```python
from build123d import *

# Parameters (mm, degrees)
SKICA1_W                 = 50
SKICA1_H                 = 50
P_IDAT_VYSUNUT_M2_DEPTH  = 3
SKICA5_W                 = 5
SKICA5_H                 = 22.5
SKICA5_W_2               = 50
SKICA5_H_2               = 5
ODEBRAT_VYSUNUT_M3_DEPTH = 1
P_IDAT_VYSUNUT_M9_DEPTH  = 15
SKICA17_R                = 2
ODEBRAT_VYSUNUT_M8_DEPTH = 4


with BuildPart() as part:
    # Skica1 → Přidat vysunutím2 (new body)
    with BuildSketch(Plane.XY):
        Rectangle(SKICA1_W, SKICA1_H)
    extrude(amount=P_IDAT_VYSUNUT_M2_DEPTH)

    # Skica5 → Odebrat vysunutím3 (cut)
    with BuildSketch(Plane(origin=(0, 0, 0), x_dir=(-1, 0, 0), z_dir=(0, 0, -1))):
        with Locations((0, -13.75)):
            Rectangle(SKICA5_W, SKICA5_H)
        Rectangle(SKICA5_W_2, SKICA5_H_2)
    extrude(amount=-ODEBRAT_VYSUNUT_M3_DEPTH, mode=Mode.SUBTRACT)

    # Skica14 → Přidat vysunutím9 (add)
    with BuildSketch(Plane.XY.offset(3)):
        Polygon((25, 25), (-25, 25), (-25, -25), (-24, -25), (-24, 24), (24, 24), (24, -25), (25, -25), align=None)
    extrude(amount=P_IDAT_VYSUNUT_M9_DEPTH)

    # Skica17 → Odebrat vysunutím8 (cut)
    with BuildSketch(Plane(origin=(0, 0, 1), x_dir=(-1, 0, 0), z_dir=(0, 0, -1))):
        with Locations((-16, 0)):
            Circle(SKICA17_R)
        with Locations((16, 0)):
            Circle(SKICA17_R)
        with Locations((0, -16)):
            Circle(SKICA17_R)
    extrude(amount=-ODEBRAT_VYSUNUT_M8_DEPTH, mode=Mode.SUBTRACT)


solid = part.part
```
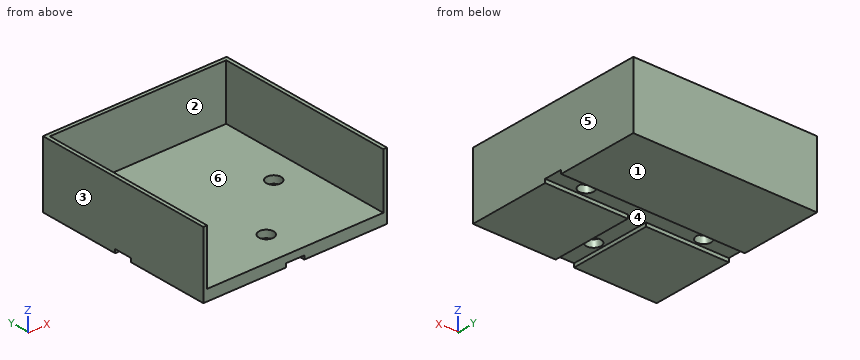
The listing builds one solid part. Answer for the finished solid, in the listing's coordinates (mm). Face numbers are marked on the shaded views. A direction names the side the tool comes from. Give positions to 0.01 mm unless a question says otherwise; leave off trailing zeros. Order: outer loops, then holes, each group sorted by start corner. A loop starts at its lowest first (then second) coordinate and runs counter-clockwise, first axis right, second up. Notation, with made-up numbers: (78.25, -13) -> (105.25, -13) arc R23 cw to (105.25, 19) -> close; hole circle Ø9 at (-6, 34.25). An arc over 180 degrees is marked (long way). Answer as a JSON object with one key per item and string values. Group by question number.
Item 1: Consider L1, parallel to X at y = 6.5, z = 6.5; L2, parallel to Y at x = 16, z = 2.6; L3, parallel to Z at x = 4, y = -2. Determine where each line is inside the solid, lowest interval first. Write a range as from..to.
Item 2: The part is cut by section D-D on y = -16. Write down the section's boundary in (x, z).
Item 3: The part is cut by section A-A on y = 0. Write down the section's boundary in (x, z).
Item 4: Flat-ended cylindrical pins translate along their axes: pin 1 (2 mm diameter, centred on x = 14.5, z = 12.5, fed in from -Y); pin 2 (0.5 mm diameter, centred on x = -1, z = 0.5, fed in from -Y); pin 3 (5 mm diameter, centred on x = 16, y = 0, fed in from +Z). Find the tip coordinate at first contact, or state that the pin passes through.
Item 5: A tool of negligible diameter and unlimited length cuts with its end or side. For the marked faces 1 and 2, from which of +Z, -Z, +X, -X, +Y, -Y can it reach the whole face along a straight path? Write none if from no direction.
Item 6: Determine the mould class of the marked faces 3, 4, 5 and 6 for opening direction X: pulls with the +X half, pulls with the -X half, needs draft (parallel to the pull), parting line crosses it, or undercut.
Item 7: The part is cut by section B-B on x = -16. Write down the section's boundary in (y, z), and give its area (3 significant figures).
Item 8: The part is cut by section C-C on z = 2.25. Write down the section's boundary in (x, y).
Result set:
{
 "1": {"L1": "-25..-24, 24..25", "L2": "-25..-2, 2..25", "L3": "1..3"},
 "2": {"outline": "(-25, 0) -> (-2.5, 0) -> (-2.5, 1) -> (-2, 1) -> (-2, 3) -> (-24, 3) -> (-24, 18) -> (-25, 18) -> close; (2, 1) -> (2.5, 1) -> (2.5, 0) -> (25, 0) -> (25, 18) -> (24, 18) -> (24, 3) -> (2, 3) -> close"},
 "3": {"outline": "(-25, 1) -> (-18, 1) -> (-18, 3) -> (-24, 3) -> (-24, 18) -> (-25, 18) -> close; (-14, 1) -> (14, 1) -> (14, 3) -> (-14, 3) -> close; (18, 1) -> (25, 1) -> (25, 18) -> (24, 18) -> (24, 3) -> (18, 3) -> close"},
 "4": {"pin 1": "y = 24", "pin 2": "y = 2.5", "pin 3": "z = 3"},
 "5": {"face 1": "-Z, +X, -X, +Y, -Y", "face 2": "+Z, -Y"},
 "6": {"face 3": "pulls with the -X half", "face 4": "undercut", "face 5": "pulls with the +X half", "face 6": "undercut"},
 "7": {"outline": "(-25, 0) -> (-2.5, 0) -> (-2.5, 1) -> (-2, 1) -> (-2, 3) -> (-25, 3) -> close; (2, 1) -> (2.5, 1) -> (2.5, 0) -> (25, 0) -> (25, 18) -> (24, 18) -> (24, 3) -> (2, 3) -> close", "area": "152 mm²"},
 "8": {"outline": "(-25, -25) -> (25, -25) -> (25, 25) -> (-25, 25) -> close; hole circle Ø4 at (-16, 0); hole circle Ø4 at (0, -16); hole circle Ø4 at (16, 0)"}
}
